For this review, take the finished solid that the model builds, in its own axes (mm). Face numbers are marked on the shaded views. A direction names the side the tool comes from. Coordinates: 2 decimals unless noted, no trailing zeros. Write each loop counter-clockwise with the first axis right and the second up, starting at its lowest first coordinate (ties: lowest second). Pieces come first, ordered by that corner, then holes. Notation, with made-up numbers: (65.5, 85) - (124.5, 85) arc R32 cw to (124.5, 113) - close; hole circle Ø11 at (42.25, -11). An arc over 180 degrees is marked (long way). Write each question's results on one line, items separated by ' | '.
from build123d import *

# Parameters (mm, degrees)
SKETCH9_R           = 145
SKETCH9_R_2         = 105
SKETCH10_W          = 360
SKETCH10_H          = 352.085339176
BOSS_EXTRUDE1_DEPTH = 50
SKETCH12_R          = 15
SKETCH12_R_2        = 105
CUT_EXTRUDE3_DEPTH  = 50
SKETCH12_3_R        = 30
CUT_EXTRUDE4_DEPTH  = 10
SKETCH19_W          = 377.161076004
SKETCH19_H          = 360
BOSS_EXTRUDE2_DEPTH = 50
SKETCH20_R          = 105
SKETCH20_R_2        = 15
CUT_EXTRUDE5_DEPTH  = 50
SKETCH20_3_R        = 30
SKETCH20_3_R_2      = 15
CUT_EXTRUDE6_DEPTH  = 10
FILLET1_R           = 10


with BuildPart() as part:
    # Sweep-Thin1: sweep along a path in Sketch1
    with BuildLine(Plane.XY) as sweep_thin1_path:
        Line((-260, 100), (-260, 0))
        ThreePointArc((-260, 0), (-183.847763109, -183.847763109), (0, -260))
        Line((0, -260), (100, -260))
    # Sketch9 → Sweep-Thin1 (sweep)
    with BuildSketch(Plane(origin=(100, 0, 0), x_dir=(0, 0, -1), z_dir=(1, 0, 0))):
        with Locations((0, -260)):
            Circle(SKETCH9_R)
        with Locations((0, -260)):
            Circle(SKETCH9_R_2, mode=Mode.SUBTRACT)
    sweep(path=sweep_thin1_path.line)

    # Sketch10 → Boss-Extrude1 (add)
    with BuildSketch(Plane(origin=(100, 0, 0), x_dir=(0, 0, -1), z_dir=(1, 0, 0))):
        with Locations((0, -260)):
            Rectangle(SKETCH10_W, SKETCH10_H)
    extrude(amount=BOSS_EXTRUDE1_DEPTH)

    # Sketch12 → Cut-Extrude3 (cut)
    with BuildSketch(Plane(origin=(150, 0, 0), x_dir=(0, 0, -1), z_dir=(1, 0, 0))):
        with Locations((-130, -133.957330412)):
            Circle(SKETCH12_R)
        with Locations((130, -133.957330412)):
            Circle(SKETCH12_R)
        with Locations((130, -393.957330412)):
            Circle(SKETCH12_R)
        with Locations((-130, -393.957330412)):
            Circle(SKETCH12_R)
        with Locations((0, -260)):
            Circle(SKETCH12_R_2)
    extrude(amount=-CUT_EXTRUDE3_DEPTH, mode=Mode.SUBTRACT)

    # Sketch12<3> → Cut-Extrude4 (cut)
    with BuildSketch(Plane(origin=(150, 0, 0), x_dir=(0, 0, -1), z_dir=(1, 0, 0))):
        with Locations((-130, -133.957330412)):
            Circle(SKETCH12_3_R)
        with Locations((130, -133.957330412)):
            Circle(SKETCH12_3_R)
        with Locations((130, -393.957330412)):
            Circle(SKETCH12_3_R)
        with Locations((-130, -393.957330412)):
            Circle(SKETCH12_3_R)
    extrude(amount=-CUT_EXTRUDE4_DEPTH, mode=Mode.SUBTRACT)

    # Sketch19 → Boss-Extrude2 (add)
    with BuildSketch(Plane(origin=(0, 100, 0), x_dir=(1, 0, 0), z_dir=(0, 1, 0))):
        with Locations((-260, 0)):
            Rectangle(SKETCH19_W, SKETCH19_H)
    extrude(amount=BOSS_EXTRUDE2_DEPTH)

    # Sketch20 → Cut-Extrude5 (cut)
    with BuildSketch(Plane(origin=(0, 150, 0), x_dir=(1, 0, 0), z_dir=(0, 1, 0))):
        with Locations(Location((-260, 0, 0), (0, 0, 180))):
            Circle(SKETCH20_R)
        with Locations(Location((-398.580538002, -130, 0), (0, 0, 270))):
            Circle(SKETCH20_R_2)
        with Locations(Location((-398.580538002, 130, 0), (0, 0, 270))):
            Circle(SKETCH20_R_2)
        with Locations(Location((-138.580538002, 130, 0), (0, 0, 270))):
            Circle(SKETCH20_R_2)
        with Locations(Location((-138.580538002, -130, 0), (0, 0, 270))):
            Circle(SKETCH20_R_2)
    extrude(amount=-CUT_EXTRUDE5_DEPTH, mode=Mode.SUBTRACT)

    # Sketch20<3> → Cut-Extrude6 (cut)
    with BuildSketch(Plane(origin=(0, 150, 0), x_dir=(1, 0, 0), z_dir=(0, 1, 0))):
        with Locations(Location((-138.580538002, -130, 0), (0, 0, 270))):
            Circle(SKETCH20_3_R)
        with Locations(Location((-138.580538002, -130, 0), (0, 0, 270))):
            Circle(SKETCH20_3_R_2, mode=Mode.SUBTRACT)
        with Locations(Location((-138.580538002, 130, 0), (0, 0, 270))):
            Circle(SKETCH20_3_R)
        with Locations(Location((-138.580538002, 130, 0), (0, 0, 270))):
            Circle(SKETCH20_3_R_2, mode=Mode.SUBTRACT)
        with Locations(Location((-398.580538002, 130, 0), (0, 0, 270))):
            Circle(SKETCH20_3_R)
        with Locations(Location((-398.580538002, 130, 0), (0, 0, 270))):
            Circle(SKETCH20_3_R_2, mode=Mode.SUBTRACT)
        with Locations(Location((-398.580538002, -130, 0), (0, 0, 270))):
            Circle(SKETCH20_3_R)
        with Locations(Location((-398.580538002, -130, 0), (0, 0, 270))):
            Circle(SKETCH20_3_R_2, mode=Mode.SUBTRACT)
    extrude(amount=-CUT_EXTRUDE6_DEPTH, mode=Mode.SUBTRACT)

    # Fillet1
    fillet1_edges = [part.edges().sort_by_distance(p)[0] for p in [
        (-155, 150, 0),
        (150, -260, 105),
    ]]
    fillet(fillet1_edges, radius=FILLET1_R)


solid = part.part
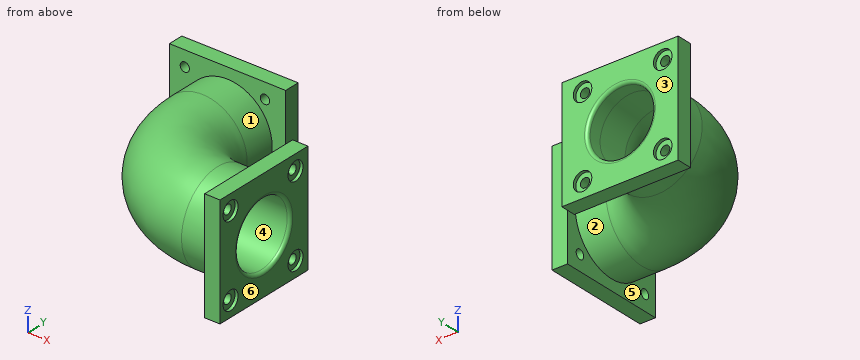
Q1. Take a section at B-B on x = 47. State the section outline as (y, z) points, plus the area to 3 significant figures.
Results found:
outline: circle Ø290 at (-260, 0); hole circle Ø210 at (-260, 0) | area: 31,400 mm2
Q2. Wall thickness on line 1 along Y through (x, z) = (113.5, 130); line 2 along X through (y, z) = (128.5, -130); line 3 along Y through (x, z) = (143.75, 130): over which ranges is each line inside the solid? List them lowest first. Write a range as from..to.
Results found:
line 1: -436.04..-408.96, -378.96..-148.96, -118.96..-83.96 | line 2: -448.58..-413.58, -383.58..-153.58, -123.58..-71.42 | line 3: -436.04..-423.96, -363.96..-163.96, -103.96..-83.96
Q3. For pin 1 (1 mm diameter, centred on y = -123.5, z = 143.5, fed in from +X); pin 2 (18 mm diameter, centred on x = -133, z = -144, fed in from +Y); pin 3 (4 mm diameter, centred on x = -380, y = 17, fed in from +Z); pin 4 (18 mm diameter, centred on y = -393.96, z = 130, fed in from -X), all flat-tipped, find the tip position at first contact; note any pin that passes through.
Results found:
pin 1: x = 140 | pin 2: y = 140 | pin 3: z = 84.27 | pin 4: through
Q4. Take a section at A-A on z = 0. State the section outline as (x, y) points.
Results found:
outline: (-448.58, 100) - (-405, 100) - (-405, 0) arc R405 ccw to (0, -405) - (100, -405) - (100, -436.04) - (150, -436.04) - (150, -375) arc R10 ccw to (140, -365) - (0, -365) arc R365 cw to (-365, 0) - (-365, 140) arc R10 ccw to (-375, 150) - (-448.58, 150) - close; (-155, 0) arc R155 ccw to (0, -155) - (140, -155) arc R10 ccw to (150, -145) - (150, -83.96) - (100, -83.96) - (100, -115) - (0, -115) arc R115 cw to (-115, 0) - (-115, 100) - (-71.42, 100) - (-71.42, 150) - (-145, 150) arc R10 ccw to (-155, 140) - close
Q5. Take a section at D-D on x = -99. State how many separate pieces and enclosed holes the cut face has, plus the area to 3 significant figures.
Results found:
separate pieces: 2 | enclosed holes: 1 | area: 54,400 mm2
Q6. Mouldability with a two-part tool opening along Y and no side actions: class the marked faces 1, 2 and 3 as pulls with the +Y half, pulls with the -Y half, needs draft (parallel to the pull), parting line crosses it, or undercut.
Results found:
face 1: undercut | face 2: parting line crosses it | face 3: pulls with the +Y half
Q7. For the marked faces 4, 5 and 6, list the 3-axis set-ups (+Z, -Z, +X, -X, +Y, -Y) from which the entire face can be reached by the end or side of a thin tool; tool diameter is ignored.
Results found:
face 4: +X | face 5: none | face 6: +Z, -Z, +X, +Y, -Y
